Build history of the part. All positions in model axes, mm. Face numbers are marked on the shaded views. A direction names the side the tool comes from. Round coordinates to 2 decimals unless told otherwise and drop trailing zeros. Write each loop counter-clockwise with the first axis right and the second up, starting at its lowest first coordinate (ties: lowest second). Pieces come first, ordered by that corner, then holes.
1) Saw through at C-C (z = 15). Write the cut outline in (x, y), plus the area to 3 significant figures.
2) Saw through at A-A (x = 50.5). Write the cut outline in (y, z).
3) Wall check: probe 1 along Y at (x, z) = (103.5, 29); probe 2 along X at (y, z) = (-8.5, 30); probe 3 along Z at (x, y) = (106.5, 75.5). Give the ranges that are in metal, low to high.
4) Which spindle directions (+Z, -Z, +X, -X, +Y, -Y) get a long thin tool onto all of the face, cutting with end or side? Do the marked faces 1 and 2. Say none if no direction does.
5) Saw through at B-B (y = -53). Write the cut outline in (x, z), plus the area to 3 significant figures.
6) Flat gauge pins, fed straight in: pin 1 (4 mm diameter, centred on y = -24, z = 6, fed in from -X); pin 2 (2.5 mm diameter, centred on x = 130.99, y = 90.5, fed in from -Z); pin 3 (3.5 mm diameter, centred on x = 131.01, y = -4, fed in from +Z). Where does each tip first touch, or does it go through?
7) Saw through at D-D (x = 125). Write the cut outline in (y, z), plus the area to 3 significant figures.
from build123d import *

# Parameters (mm, degrees)
EXTRUDE_1_DEPTH     = 8
CUT_EXTRUDE_1_DEPTH = 2
SKETCH_3_R          = 2
CUT_EXTRUDE_2_DEPTH = 5
SKETCH_4_W          = 8
SKETCH_4_H          = 97.5
EXTRUDE_2_DEPTH     = 60
FILLET_1_R          = 2
SKETCH_5_W          = 70
SKETCH_5_H          = 24.5
CUT_EXTRUDE_4_DEPTH = 20


with BuildPart() as part:
    # 스케치1 → 보스-돌출1 (new body)
    with BuildSketch(Plane.XY):
        Polygon((0, 0), (70, 0), (70, 97.5), (140, 97.5), (140, -19.573170732), (140, -97.5), (0, -97.5), align=None)
    extrude(amount=EXTRUDE_1_DEPTH)

    # 스케치2 → 컷-돌출1 (cut)
    with BuildSketch(Plane.XY):
        Polygon((127.5, 90.5), (129.25, 87.468911087), (132.75, 87.468911087), (134.5, 90.5), (132.75, 93.531088913), (129.25, 93.531088913), align=None)
        Polygon((129.25, -7.031088913), (132.75, -7.031088913), (134.5, -4), (132.75, -0.968911087), (129.25, -0.968911087), (127.5, -4), align=None)
        Polygon((136.5, -87.08), (134.75, -84.048911087), (131.25, -84.048911087), (129.5, -87.08), (131.25, -90.111088913), (134.75, -90.111088913), align=None)
        Polygon((83.25, -77.468911087), (81.5, -80.5), (83.25, -83.531088913), (86.75, -83.531088913), (88.5, -80.5), (86.75, -77.468911087), align=None)
        Polygon((83.25, -87.468911087), (81.5, -90.5), (83.25, -93.531088913), (86.75, -93.531088913), (88.5, -90.5), (86.75, -87.468911087), align=None)
        Polygon((37.25, -7.001775013), (40.75, -7.001775013), (42.5, -3.9706861), (40.75, -0.939597187), (37.25, -0.939597187), (35.5, -3.9706861), align=None)
    extrude(amount=CUT_EXTRUDE_1_DEPTH, mode=Mode.SUBTRACT)

    # 스케치3 → 컷-돌출2 (cut)
    with BuildSketch(Plane.XY.offset(2)):
        with Locations((130.98963708, 90.501088913)):
            Circle(SKETCH_3_R)
        with Locations((131.01036292, -3.998911087)):
            Circle(SKETCH_3_R)
        with Locations((39.010362751, -3.969597187)):
            Circle(SKETCH_3_R)
        with Locations((85.01036292, -80.498911087)):
            Circle(SKETCH_3_R)
        with Locations((84.989637249, -90.501088913)):
            Circle(SKETCH_3_R)
        with Locations((132.98963708, -87.078911087)):
            Circle(SKETCH_3_R)
    extrude(amount=CUT_EXTRUDE_2_DEPTH, mode=Mode.SUBTRACT)

    # 스케치4 → 보스-돌출2 (add)
    with BuildSketch(Plane.XY.offset(8)):
        with Locations((136, -40.75)):
            Rectangle(SKETCH_4_W, SKETCH_4_H)
        Polygon((70, -97.5), (140, -97.5), (140, -89.5), (132, -89.5), (70, -89.5), align=None)
    extrude(amount=EXTRUDE_2_DEPTH)

    # 필렛1
    fillet_1_edges = [part.edges().sort_by_distance(p)[0] for p in [
        (140, -97.5, 34),
        (140, 52.75, 8),
        (132, -40.75, 68),
        (132, -89.5, 38),
        (70, -93.5, 68),
        (70, -97.5, 38),
        (140, 8, 38),
        (101, -89.5, 68),
        (105, -97.5, 68),
        (140, -44.75, 68),
        (136, 8, 68),
        (35, -97.5, 8),
    ]]
    fillet(fillet_1_edges, radius=FILLET_1_R)

    # 스케치5 → 컷-돌출4 (cut)
    with BuildSketch(Plane.XY.offset(8)):
        with Locations((35, -27.25)):
            Rectangle(SKETCH_5_W, SKETCH_5_H)
    extrude(amount=-CUT_EXTRUDE_4_DEPTH, mode=Mode.SUBTRACT)


solid = part.part
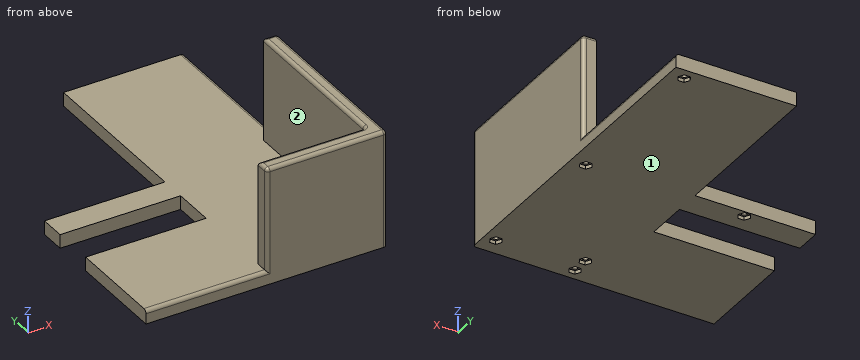
Evaluation:
1. outline: (70, -95.5) arc R2 ccw to (72, -97.5) - (138, -97.5) arc R2 ccw to (140, -95.5) - (140, 6) arc R2 ccw to (138, 8) - (132, 8) - (132, -87.5) arc R2 cw to (130, -89.5) - (70, -89.5) - close
1. area: 1,340 mm2
2. outline: (-97.5, 0) - (-39.5, 0) - (-39.5, 8) - (-95.5, 8) arc R2 ccw to (-97.5, 6) - close; (-15, 0) - (0, 0) - (0, 8) - (-15, 8) - close
3. probe 1: y = -97.5 to -89.5
3. probe 2: x = 132 to 140
3. probe 3: z = 0 to 8
4. face 1: -Z, +X, -X, +Y, -Y
4. face 2: +Z, -X, +Y
5. outline: (0, 0) - (140, 0) - (140, 66) arc R2 ccw to (138, 68) - (134, 68) arc R2 ccw to (132, 66) - (132, 8) - (0, 8) - close
5. area: 1,600 mm2
6. pin 1: stops at x = 70
6. pin 2: stops at z = 7
6. pin 3: stops at z = 67.57
7. outline: (-97.5, 0) - (97.5, 0) - (97.5, 8) - (-89.5, 8) - (-89.5, 66) arc R2 ccw to (-91.5, 68) - (-95.5, 68) arc R2 ccw to (-97.5, 66) - close
7. area: 2,040 mm2
